Verification items for the finished model (mm, model axes). A direction names the side the tool comes from. Give positions to 0.01 mm unless a question says otherwise; leave off trailing zeros. Loops run counter-clockwise (first coordinate to the right, second up) from the corner with the lowest first, then second, coordinate; pieces in that order, holes last. Notation, with made-up numbers: M 2,88.25 L 57,88.25 A35 ccw 57,120.25 Z; hole C 26.25,-1.5 d11. An arc over 180 degrees is marked long. Use a Markdown table: item, result.
from build123d import *

# Parameters (mm, degrees)
SKETCH_W        = 54.3
SKETCH_H        = 38.5
PAD_DEPTH       = 2
SKETCH003_W     = 6.85
SKETCH003_H     = 15
PAD001_DEPTH    = 20
SKETCH001_W     = 54.3
SKETCH001_H     = 2
PAD003_DEPTH    = 32
SKETCH005_W     = 6.85
SKETCH005_H     = 15
PAD004_DEPTH    = 20
SKETCH002_R     = 2.45
PAD005_DEPTH    = 5
SKETCH007_W     = 25
SKETCH007_H     = 32
PAD006_DEPTH    = 2
SKETCH006_R     = 1.5
POCKET_DEPTH    = 15
SKETCH004_R     = 1.5
POCKET001_DEPTH = 20
SKETCH009_R     = 1.5
SKETCH009_R_2   = 2.95
POCKET002_DEPTH = 2
SKETCH008_R     = 1.5
POCKET003_DEPTH = 3
SKETCH010_W     = 42.5
SKETCH010_H     = 32
PAD007_DEPTH    = 2
FILLET_R        = 1.8
FILLET001_R     = 1.8
FILLET002_R     = 1.8
FILLET003_R     = 3


with BuildPart() as part:
    # Sketch → Pad (new body)
    with BuildSketch(Plane.XY):
        with Locations((27.15, 21.25)):
            Rectangle(SKETCH_W, SKETCH_H)
    extrude(amount=PAD_DEPTH)

    # Sketch003 → Pad001 (join)
    with BuildSketch(Plane.XY.offset(2)):
        with Locations((3.425, 20.3)):
            Rectangle(SKETCH003_W, SKETCH003_H)
    extrude(amount=PAD001_DEPTH)

    # Sketch001 → Pad003 (join)
    with BuildSketch(Plane.XY):
        with Locations((27.15, 1)):
            Rectangle(SKETCH001_W, SKETCH001_H)
    extrude(amount=PAD003_DEPTH)

    # Sketch005 (on Face5 of Pad003) → Pad004 (join)
    with BuildSketch(Plane.XY.offset(2)):
        with Locations((50.875, 20.3)):
            Rectangle(SKETCH005_W, SKETCH005_H)
    extrude(amount=PAD004_DEPTH)

    # Sketch002 (on Face18 of Pad004) → Pad005 (join)
    with BuildSketch(Plane.XZ):
        with Locations((37.25, 12)):
            Circle(SKETCH002_R)
    extrude(amount=PAD005_DEPTH)

    # Sketch007 (on Face1 of Pad005) → Pad006 (join)
    with BuildSketch(Plane(origin=(0, 40.5, 0), x_dir=(-1, 0, 0), z_dir=(0, 1, 0))):
        with Locations((-12.5, 16)):
            Rectangle(SKETCH007_W, SKETCH007_H)
    extrude(amount=PAD006_DEPTH)

    # Sketch006 (on Face14 of Pad006) → Pocket (cut)
    with BuildSketch(Plane.XZ.offset(-12.8)):
        with Locations((51.3, 17)):
            Circle(SKETCH006_R)
        with Locations((51.3, 7)):
            Circle(SKETCH006_R)
    extrude(amount=-POCKET_DEPTH, mode=Mode.SUBTRACT)

    # Sketch004 (on Face16 of Pocket) → Pocket001 (cut)
    with BuildSketch(Plane.XZ.offset(-12.8)):
        with Locations((3, 17)):
            Circle(SKETCH004_R)
        with Locations((3, 7)):
            Circle(SKETCH004_R)
    extrude(amount=-POCKET001_DEPTH, mode=Mode.SUBTRACT)

    # Sketch009 (on Face20 of Pocket001) → Pocket002 (cut)
    with BuildSketch(Plane(origin=(0, 42.5, 0), x_dir=(-1, 0, 0), z_dir=(0, 1, 0))):
        with Locations((-6, 25)):
            Circle(SKETCH009_R)
        with Locations((-19, 25)):
            Circle(SKETCH009_R)
        with Locations((-3, 7)):
            Circle(SKETCH009_R_2)
        with Locations((-3, 17)):
            Circle(SKETCH009_R_2)
    extrude(amount=-POCKET002_DEPTH, mode=Mode.SUBTRACT)

    # Sketch008 → Pocket003 (cut)
    with BuildSketch(Plane.XZ):
        with Locations((19, 25)):
            Circle(SKETCH008_R)
        with Locations((6, 25)):
            Circle(SKETCH008_R)
    extrude(amount=-POCKET003_DEPTH, mode=Mode.SUBTRACT)

    # Sketch010 (on Face8 of Pocket003) → Pad007 (join)
    with BuildSketch(Plane(origin=(0, 0, 0), x_dir=(0, -1, 0), z_dir=(-1, 0, 0))):
        with Locations((-21.25, 16)):
            Rectangle(SKETCH010_W, SKETCH010_H)
    extrude(amount=PAD007_DEPTH)

    # Fillet
    fillet_edges = [part.edges().sort_by_distance(p)[0] for p in [
        (-2, 42.5, 16),
    ]]
    fillet(fillet_edges, radius=FILLET_R)

    # Fillet001
    fillet001_edges = [part.edges().sort_by_distance(p)[0] for p in [
        (-2, 0, 16),
    ]]
    fillet(fillet001_edges, radius=FILLET001_R)

    # Fillet002
    fillet002_edges = [part.edges().sort_by_distance(p)[0] for p in [
        (-2, 21.25, 0),
    ]]
    fillet(fillet002_edges, radius=FILLET002_R)

    # Fillet003
    fillet003_edges = [part.edges().sort_by_distance(p)[0] for p in [
        (54.3, 20.3, 22),
    ]]
    fillet(fillet003_edges, radius=FILLET003_R)


solid = part.part
(1) Gauge pin test, flat ends, axial feed: P1, Ø1.9, axis at x = 48.5, y = 17.5, coming from the +Z side; P2, Ø1.5, axis at x = 43, z = 23.5, coming from the +Y side; P3, Ø1.5, axis at x = 15.5, z = 7.5, coming from the -Y side; P4, Ø2.5, axis at x = 6, z = 25, coming from the +Y side. Record the tip position at first contact, or that the pin passes through.
Results below:
| item | result |
|---|---|
| P1 | z = 22 |
| P2 | y = 2 |
| P3 | y = 0 |
| P4 | through |
(2) Cross-section at C-C on x = 3. State how many separate pieces and enclosed holes the cut face has, then the cut area to 3 significant figures.
Results below:
| item | result |
|---|---|
| separate pieces | 5 |
| enclosed holes | 0 |
| area | 390 mm^2 |
(3) Cross-section at A-A on z = 25. Record the cut outline in (x, y), then the cut area to 3 significant figures.
Results below:
| item | result |
|---|---|
| outline | M -2,1.8 A1.8 ccw -0.2,0 L 4.5,0 L 4.5,2 L 0,2 L 0,40.5 L 4.5,40.5 L 4.5,42.5 L -0.2,42.5 A1.8 ccw -2,40.7 Z; M 7.5,0 L 17.5,0 L 17.5,2 L 7.5,2 Z; M 7.5,40.5 L 17.5,40.5 L 17.5,42.5 L 7.5,42.5 Z; M 20.5,0 L 54.3,0 L 54.3,2 L 20.5,2 Z; M 20.5,40.5 L 25,40.5 L 25,42.5 L 20.5,42.5 Z |
| area | 218 mm^2 |
(4) Set-up check for faces 4 (the flat face through (3, 27.8, 12)), 5 (the cylindrical face through (52.73, 20.2, 17.45)), 6 (the flat face through (6.85, 20, 12)): record each of +Z, -Z, +X, -X, +Y, -Y from which the full face is reachable in a straight line by a thin tool's end or side.
Results below:
| item | result |
|---|---|
| face 4 | +Z, +X |
| face 5 | +Y |
| face 6 | +Z |
(5) Material ranges on line 1 (Y direction, x = 3.5, z = 10); line 2 (Z direction, x = 19, y = 1.4) (3 decimals); line 3 (Y direction, x = 49, z = 12.5), recorded low to high.
Results below:
| item | result |
|---|---|
| line 1 | 0 to 2, 12.8 to 27.8, 40.5 to 42.5 |
| line 2 | 0.045 to 23.5, 26.5 to 32 |
| line 3 | 0 to 2, 12.8 to 27.8 |
(6) Cross-section at B-B on y = 21. Record the cut outline in (x, z).
Results below:
| item | result |
|---|---|
| outline | M -2,1.8 A1.8 ccw -0.2,0 L 54.3,0 L 54.3,19 A3 ccw 51.3,22 L 47.45,22 L 47.45,2 L 6.85,2 L 6.85,22 L 0,22 L 0,32 L -2,32 Z; hole C 3,7 d3; hole C 3,17 d3; hole C 51.3,7 d3; hole C 51.3,17 d3 |
(7) Draft check along Z on faces 1 (the cylindrical face through (53.44, 20.4, 21.1)), 2 (the cylindrical face through (5.174, 41.514, 8.994)), 3 (the cylindrical face through (-1.459, 41.987, 17.111)). Enter one of: +Z half, -Z half, draft (parallel to the pull), parting line (faces both ways), or undercut.
Results below:
| item | result |
|---|---|
| face 1 | +Z half |
| face 2 | undercut |
| face 3 | draft |
(8) Cross-section at D-D on z = 12. Record the cut outline in (x, y).
Results below:
| item | result |
|---|---|
| outline | M -2,1.8 A1.8 ccw -0.2,0 L 34.8,0 L 34.8,-5 L 39.7,-5 L 39.7,0 L 54.3,0 L 54.3,2 L 0,2 L 0,12.8 L 6.85,12.8 L 6.85,27.8 L 0,27.8 L 0,40.5 L 25,40.5 L 25,42.5 L -0.2,42.5 A1.8 ccw -2,40.7 Z; M 47.45,12.8 L 54.3,12.8 L 54.3,27.8 L 47.45,27.8 Z |
